```python
from build123d import *

# Parameters (mm, degrees)
F0_R     = 7.25
F1_DEPTH = 5
F0_R_2   = 6.5
F2_DEPTH = 1
F4_DEPTH = 3


with BuildPart() as f1:
    # F0 (on Top) → F1 (new body)
    with BuildSketch(Plane.XY):
        with BuildLine():
            Line((20, 9), (0, 9))
            ThreePointArc((0, 9), (-9, 0), (0, -9))
            Line((0, -9), (20, -9))
            ThreePointArc((20, -9), (29, 0), (20, 9))
        make_face()
        Circle(F0_R, mode=Mode.SUBTRACT)
    extrude(amount=F1_DEPTH)

    # F0 (on Top) → F2 (join)
    with BuildSketch(Plane.XY):
        Circle(F0_R)
        Circle(F0_R_2, mode=Mode.SUBTRACT)
    extrude(amount=F2_DEPTH)

    # F3 (on face) → F4 (cut)
    with BuildSketch(Plane.XY.offset(5)):
        with BuildLine():
            ThreePointArc((0, 9), (9, 0), (0, -9))
            Line((0, -9), (20, -9))
            ThreePointArc((20, -9), (29, 0), (20, 9))
            Line((20, 9), (0, 9))
        make_face()
    extrude(amount=-F4_DEPTH, mode=Mode.SUBTRACT)


solid = f1.part
```
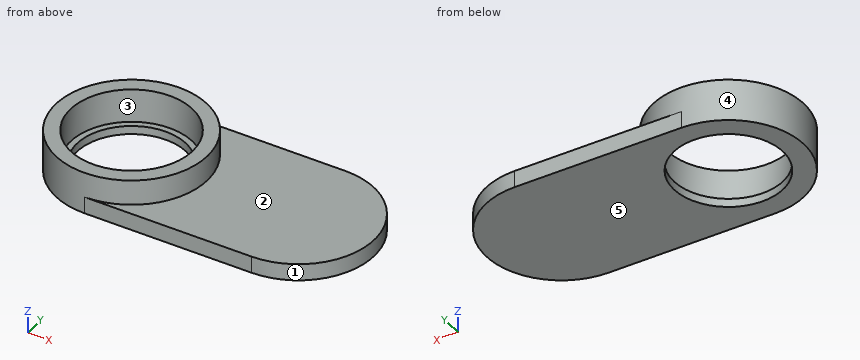
Can you work these out from the model? Positions are in its coordinate system, mm. Face numbers are marked on the shaded views. A direction names the side the tool comes from. Give positions to 0.01 mm unless a question says otherwise; leave off trailing zeros. Write each loop counter-clockwise with the first axis right and the second up, starting at its lowest first coordinate (ties: lowest second). Pieces come first, ordered by that corner, then holes. Notation, with made-up numbers: (61, -35) -> (91, -35) arc R32 cw to (91, -2) -> close; hole circle Ø2 at (55, -34.75). An arc over 180 degrees is marked (long way). Write item = value, one per line.
(1) Thinking about a two-plate mould opening in X: for the marked faces 1, 2 and 3, which applies, released by +X, released by -X, zero draft, split by the parting line, or undercut?
Worked out:
face_1 = released by +X
face_2 = zero draft
face_3 = undercut
(2) Suppose I cut it at C-C on x = 5. Write out the boundary of the cut face in (y, z), then the cut area to 3 significant figures.
Worked out:
outline = (-9, 0) -> (-4.15, 0) -> (-4.15, 1) -> (-5.25, 1) -> (-5.25, 5) -> (-7.48, 5) -> (-7.48, 2) -> (-9, 2) -> close; (4.15, 0) -> (9, 0) -> (9, 2) -> (7.48, 2) -> (7.48, 5) -> (5.25, 5) -> (5.25, 1) -> (4.15, 1) -> close
area = 30.6 mm^2
(3) I need wall thicknesses on probe 1 along Y at (x, z) = (0, 0.3); probe 2 along Y at (x, z) = (0, 1.9); probe 3 along Z at (x, y) = (27.5, 2). Which ranges of each line are inside material? Lowest first, please. Write a range as from..to.
Worked out:
probe_1 = -9..-6.5, 6.5..9
probe_2 = -9..-7.25, 7.25..9
probe_3 = 0..2
(4) For the marked faces 4 and 5, which set-ups out of +Z, -Z, +X, -X, +Y, -Y let a thin tool reach every point of the face, with its end or its side?
Worked out:
face_4 = +Z
face_5 = -Z, +X, -X, +Y, -Y
(5) I'm going to push a flat-ended pin straight in: P1, Ø1.5, axis at x = 25, y = -1, coming from the +Z side. Where does the tip first touch, or does it pass through?
Worked out:
P1 = 2
(6) Suppose I cut it at A-A on y = 0. Write out the boundary of the cut face in (x, z).
Worked out:
outline = (-9, 0) -> (-6.5, 0) -> (-6.5, 1) -> (-7.25, 1) -> (-7.25, 5) -> (-9, 5) -> close; (6.5, 0) -> (29, 0) -> (29, 2) -> (9, 2) -> (9, 5) -> (7.25, 5) -> (7.25, 1) -> (6.5, 1) -> close
(7) Suppose I cut it at D-D on y = -5.75. Write out the boundary of the cut face in (x, z), then the cut area to 3 significant figures.
Worked out:
outline = (-6.92, 0) -> (-3.03, 0) -> (-3.03, 1) -> (-4.42, 1) -> (-4.42, 5) -> (-6.92, 5) -> close; (3.03, 0) -> (26.92, 0) -> (26.92, 2) -> (6.92, 2) -> (6.92, 5) -> (4.42, 5) -> (4.42, 1) -> (3.03, 1) -> close
area = 67.8 mm^2
(8) Suppose I cut it at B-B on z = 1.5. Write out the boundary of the cut face in (x, y), then the cut area to 3 significant figures.
Worked out:
outline = (0, -9) -> (20, -9) arc R9 ccw to (20, 9) -> (0, 9) arc R9 ccw to start; hole circle Ø14.5 at (0, 0)
area = 449 mm^2
